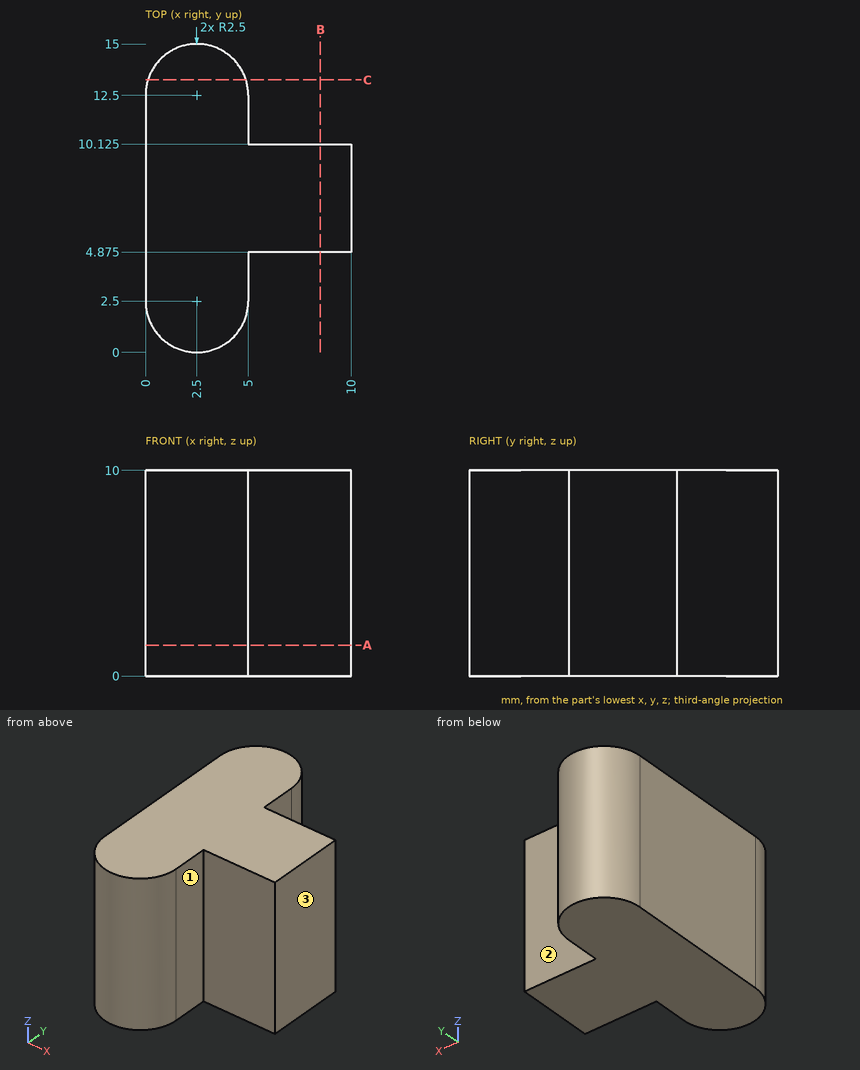
Source: three-view drawing plus pictorial views. Frame: mm from the lowest corner of the part. A direction names the side the tool comes from. Coordinates: 2 decimals unless noted, no trailing zeros. Loops run counter-clockwise (first coordinate to the right, second up) from the corner with the lowest first, then second, coordinate; pieces in that order, holes last. Notation, with made-up numbers: (44, -36.75) -> (74, -36.75) arc R17 cw to (74, -30.75) -> close; hole circle Ø9 at (11, 48). An arc over 180 degrees is marked (long way). Write each question's results on one line, items separated by ' | '. Start each with the question number.
Q1. Ray query, line 1 (Y direction, x = 8.5, z = 1.75) (3 decimals); line 2 (X direction, y = 4.75, z = 8); line 3 (X direction, y = 14.5, z = 1). Return the intervals inside material, ascending. Write a range as from..to.
Q2. Section A-A, the plane z = 1.5. Return the cut outline in (x, y) (3 decimals).
Q3. Section B-B, the plane x = 8.5. Return the cut outline in (y, z) (3 decimals), plus the area to 3 significant figures.
Q4. Pin query (flat end, axial travel): pin 1 (5 mm diameter, centred on x = 5.5, z = 7, fed in from +Y); pin 2 (2.5 mm diameter, centred on y = 11.5, z = 5.5, fed in from +X); pin 3 (5.5 mm diameter, centred on x = 6.5, z = 7.5, fed in from +Y). Return the tip coordinate at first contact, or that it passes through.
Q5. Reachability of the marked faces 1, 2 and 3 from +Z, -Z, +X, -X, +Y, -Y: full face, straight path, thin tool, end or side. Return the list, or none.
Q6. Section C-C, the plane y = 13.25. Return the cut outline in (x, z).
Found:
1) line 1: 4.875..10.125 | line 2: 0..5 | line 3: 1..4
2) outline: (0, 2.5) arc R2.5 ccw to (5, 2.5) -> (5, 4.875) -> (10, 4.875) -> (10, 10.125) -> (5, 10.125) -> (5, 12.5) arc R2.5 ccw to (0, 12.5) -> close
3) outline: (4.875, 0) -> (10.125, 0) -> (10.125, 10) -> (4.875, 10) -> close | area: 52.5 mm2
4) pin 1: y = 14.95 | pin 2: x = 5 | pin 3: y = 14.67
5) face 1: +Z, -Z, +X, -Y | face 2: +Z, -Z, +X, +Y | face 3: +Z, -Z, +X, +Y, -Y
6) outline: (0.12, 0) -> (4.88, 0) -> (4.88, 10) -> (0.12, 10) -> close
